Could you check a few things on this model? Use its own coordinates, in mm. A direction names the side the tool comes from. Coordinates: 2 decimals unless noted, no trailing zeros. Write each loop counter-clockwise with the first axis right and the second up, starting at its lowest first coordinate (ties: lowest second). Pieces come first, ordered by that corner, then holes. Notation, with made-up numbers: (66.5, 21.25) - (87.5, 21.25) arc R13 ccw to (87.5, 25.25) - close; hole circle Ø7 at (26, 43.5). An arc over 180 degrees is marked (long way). Answer as a JSON object with one key per item and string values. Group by question number.
1) If we section it at A-A (x = -16): Write out the boundary of the cut face in (y, z).
2) We'd pull the mould along Z, two halves only. Please class faces 1 (the cylindrical face through (-68.1, 16.66, 16.35)), 2 (the flat face through (-38, 11, 0)), 3 (the flat face through (-62, 20, 12.697)): released by +Z, released by -Z, zero draft, split by the parting line, or undercut.
3) If we section it at D-D (y = 40.5): Write out the boundary of the cut face in (x, z).
4) On a 3-axis mill with a long thin cutter (end or side, diameter ignored), from which of +Z, -Z, +X, -X, +Y, -Y can I reach the whole of each face in a straight line? I mean faces 4 (the flat face through (-46.218, 16.395, 18.158)), 5 (the flat face through (21, 11, 11)), 6 (the flat face through (28, 28, 5)). Say none if no direction works.
5) If we section it at C-C (z = -5): Write out the boundary of the cut face in (x, y), plus the area to 3 significant figures.
6) Will these pins go through, and if not, where does the flat tip stop? pin 1 Ø7 at (y, z) = (16, 18.5) entering from -X; pin 2 Ø3 at (x, y) = (20, 21.5) entering from -Z; pin 3 Ø15 at (x, y) = (21.5, 35) entering from +Z.
7) Please list where these lines run through material, in increasing order: line 1 along X through (y, z) = (9.5, 4); line 2 along Z through (x, y) = (11, 36); line 3 along X through (y, z) = (34, 4.5).
8) If we section it at B-B (y = 18): Write out the boundary of the cut face in (x, z).
```python
from build123d import *

# Parameters (mm, degrees)
SKETCH_1_W          = 162
SKETCH_1_H          = 53
EXTRUDE_1_DEPTH     = 9
EXTRUDE_2_DEPTH     = 15
SKETCH_5_W          = 39.196939595
SKETCH_5_H          = 7.5
CUT_EXTRUDE_1_DEPTH = 157.5
SKETCH_6_R          = 3.25
CUT_EXTRUDE_2_DEPTH = 15
SKETCH_7_W          = 119
SKETCH_7_H          = 22
EXTRUDE_3_DEPTH     = 4
SKETCH_8_W          = 18.5
SKETCH_8_H          = 3
EXTRUDE_4_DEPTH     = 30


with BuildPart() as part:
    # 草图1 → 凸台-拉伸1 (new body)
    with BuildSketch(Plane(origin=(0, 0, 0), x_dir=(1, 0, 0), z_dir=(0, 1, 0))):
        Rectangle(SKETCH_1_W, SKETCH_1_H)
    extrude(amount=EXTRUDE_1_DEPTH)

    # 草图2 → 凸台-拉伸2 (add)
    with BuildSketch(Plane(origin=(0, 9, 0), x_dir=(1, 0, 0), z_dir=(0, 1, 0))):
        Polygon((-75.5, 26.5), (-75.5, -26.5), (-44, -26.5), (-44, -20.5), (-48.5, -15.75), (-48.5, 15.75), (-44, 20.5), (-44, 26.5), align=None)
    extrude(amount=EXTRUDE_2_DEPTH)

    # 草图5 → 切除-拉伸1 (cut, through all)
    with BuildSketch(Plane.ZY.offset(75.5)):
        with Locations((-6.901530203, 20.25)):
            Rectangle(SKETCH_5_W, SKETCH_5_H)
    extrude(amount=-CUT_EXTRUDE_1_DEPTH, mode=Mode.SUBTRACT)

    # 草图6 → 切除-拉伸2 (cut)
    with BuildSketch(Plane.ZY.offset(75.5)):
        with Locations((19.598469797, 16.517563147)):
            Circle(SKETCH_6_R)
    extrude(amount=-CUT_EXTRUDE_2_DEPTH, mode=Mode.SUBTRACT)

    # 草图7 → 凸台-拉伸3 (add)
    with BuildSketch(Plane(origin=(0, 9, 0), x_dir=(1, 0, 0), z_dir=(0, 1, 0))):
        with Locations((21.5, 0)):
            Rectangle(SKETCH_7_W, SKETCH_7_H)
    extrude(amount=EXTRUDE_3_DEPTH)

    # 草图8 → 凸台-拉伸4 (add)
    with BuildSketch(Plane(origin=(0, 13, 0), x_dir=(1, 0, 0), z_dir=(0, 1, 0))):
        with Locations((18.75, -5)):
            Rectangle(SKETCH_8_W, SKETCH_8_H)
    extrude(amount=EXTRUDE_4_DEPTH)


solid = part.part
```
Here are the results:
{
 "1": {"outline": "(0, -26.5) - (9, -26.5) - (9, -11) - (13, -11) - (13, 11) - (9, 11) - (9, 26.5) - (0, 26.5) - close"},
 "2": {"face 1": "undercut", "face 2": "zero draft", "face 3": "released by -Z"},
 "3": {"outline": "(9.5, 3.5) - (28, 3.5) - (28, 6.5) - (9.5, 6.5) - close"},
 "4": {"face 4": "+X, +Y", "face 5": "+Z, +X, +Y", "face 6": "+Z, -Z, +X, +Y"},
 "5": {"outline": "(-81, 0) - (81, 0) - (81, 13) - (-38, 13) - (-38, 9) - (-48.5, 9) - (-48.5, 16.5) - (-75.5, 16.5) - (-75.5, 9) - (-81, 9) - close", "area": "2,140 mm²"},
 "6": {"pin 1": "stops at x = -75.5", "pin 2": "stops at z = 3.5", "pin 3": "stops at z = 6.5"},
 "7": {"line 1": "x = -75.5 to -48.5, -38 to 81", "line 2": "z = 3.5 to 6.5", "line 3": "x = 9.5 to 28"},
 "8": {"outline": "(-75.5, 12.7) - (-48.5, 12.7) - (-48.5, 15.75) - (-44, 20.5) - (-44, 26.5) - (-75.5, 26.5) - (-75.5, 22.49) - (-60.5, 22.49) - (-60.5, 16.71) - (-75.5, 16.71) - close; (9.5, 3.5) - (28, 3.5) - (28, 6.5) - (9.5, 6.5) - close"}
}
